Check sheet for the modelled part. Datum: model origin and axes. Units: mm. Face numbers are marked on the shaded views. A direction names the side the tool comes from. Round coordinates to 2 decimals unless told otherwise and drop trailing zeros. Write each loop counter-clockwise with the first axis right and the second up, starting at its lowest first coordinate (ties: lowest second). Pieces come first, ordered by that corner, then holes. Notation, with made-up numbers: (-26, 64) -> (-9, 64) arc R25 ccw to (-9, 82) -> close; hole circle Ø8 at (77.5, 32). An arc over 180 degrees is marked (long way). Answer as a JSON object with one key per item and string values. Group by question number.
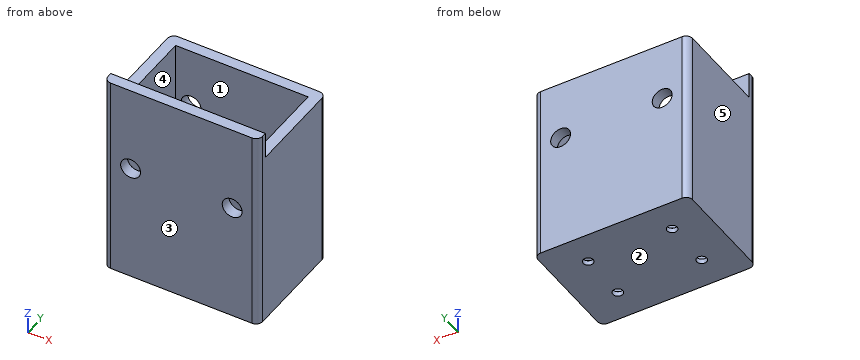
```python
from build123d import *

# Parameters (mm, degrees)
SKETCH1_W                                   = 70
SKETCH1_H                                   = 50
BOSS_EXTRUDE1_DEPTH                         = 5
SKETCH2_W                                   = 70
SKETCH2_H                                   = 5
BOSS_EXTRUDE2_DEPTH                         = 88
BOSS_EXTRUDE3_DEPTH                         = 76
SKETCH4_R                                   = 4.5
CUT_EXTRUDE1_DEPTH                          = 56
FILLET1_R                                   = 3
CBORE_FOR_M4_HEX_HEAD_CAP_SCREW1_AT_2_COUNT = 2
CBORE_FOR_M4_HEX_HEAD_CAP_SCREW1_AT_2_PITCH = 22
CBORE_FOR_M4_HEX_HEAD_CAP_SCREW1_AT_3_COUNT = 2
CBORE_FOR_M4_HEX_HEAD_CAP_SCREW1_AT_3_PITCH = 43.9089968
CBORE_FOR_M4_HEX_HEAD_CAP_SCREW1_AT_4_COUNT = 2
CBORE_FOR_M4_HEX_HEAD_CAP_SCREW1_AT_4_PITCH = 38


with BuildPart() as part:
    # Sketch1 → Boss-Extrude1 (new body)
    with BuildSketch(Plane.XY):
        Rectangle(SKETCH1_W, SKETCH1_H)
    extrude(amount=BOSS_EXTRUDE1_DEPTH)

    # Sketch2 → Boss-Extrude2 (add)
    with BuildSketch(Plane.XY.offset(5)):
        with Locations((0, -22.5)):
            Rectangle(SKETCH2_W, SKETCH2_H)
    extrude(amount=BOSS_EXTRUDE2_DEPTH)

    # Sketch3 → Boss-Extrude3 (add)
    with BuildSketch(Plane.XY.offset(5)):
        Polygon((-35, 25), (35, 25), (35, 20), (35, -20), (30, -20), (30, 20), (-30, 20), (-30, -20), (-35, -20), (-35, 20), align=None)
    extrude(amount=BOSS_EXTRUDE3_DEPTH)

    # Sketch4 → Cut-Extrude1 (cut)
    with BuildSketch(Plane(origin=(0, 25, 0), x_dir=(1, 0, 0), z_dir=(0, 1, 0))):
        with Locations(Location((23, -54, 0), (0, 0, 270))):
            Circle(SKETCH4_R)
        with Locations(Location((-23, -54, 0), (0, 0, 270))):
            Circle(SKETCH4_R)
    extrude(amount=-CUT_EXTRUDE1_DEPTH, mode=Mode.SUBTRACT)

    # Fillet1
    fillet1_edges = [part.edges().sort_by_distance(p)[0] for p in [
        (-35, 25, 40.5),
        (35, 25, 40.5),
        (35, -25, 46.5),
        (-35, -25, 46.5),
    ]]
    fillet(fillet1_edges, radius=FILLET1_R)

    # Sketch7 → CBORE for M4 Hex Head Cap Screw1 (revolve, cut)
    with BuildSketch(Plane(origin=(-19, -11, 5), x_dir=(0, -1, 0), z_dir=(1, 0, 0))):
        Polygon((0, 0), (0, 12.4), (2.25, 11.048063607), (2.25, 2.8), (5.5415, 2.8), (5.5415, 0.025), (5.5665, 0), align=None)
    cbore_for_m4_hex_head_cap_screw1 = revolve(axis=Axis((-19, -11, 11.35), (0, 0, -1)), mode=Mode.SUBTRACT)

    # CBORE for M4 Hex Head Cap Screw1 at 2: CBORE for M4 Hex Head Cap Screw1 ×2
    with Locations(*[(0, i * CBORE_FOR_M4_HEX_HEAD_CAP_SCREW1_AT_2_PITCH, 0) for i in range(1, CBORE_FOR_M4_HEX_HEAD_CAP_SCREW1_AT_2_COUNT)]):
        add(cbore_for_m4_hex_head_cap_screw1, mode=Mode.SUBTRACT)

    # CBORE for M4 Hex Head Cap Screw1 at 3: CBORE for M4 Hex Head Cap Screw1 ×2
    with Locations(*[Vector(0.8654262854811263, 0.5010362705417046, 0) * (i * CBORE_FOR_M4_HEX_HEAD_CAP_SCREW1_AT_3_PITCH) for i in range(1, CBORE_FOR_M4_HEX_HEAD_CAP_SCREW1_AT_3_COUNT)]):
        add(cbore_for_m4_hex_head_cap_screw1, mode=Mode.SUBTRACT)

    # CBORE for M4 Hex Head Cap Screw1 at 4: CBORE for M4 Hex Head Cap Screw1 ×2
    with Locations(*[(i * CBORE_FOR_M4_HEX_HEAD_CAP_SCREW1_AT_4_PITCH, 0, 0) for i in range(1, CBORE_FOR_M4_HEX_HEAD_CAP_SCREW1_AT_4_COUNT)]):
        add(cbore_for_m4_hex_head_cap_screw1, mode=Mode.SUBTRACT)


solid = part.part
```
(1) Go/stop test with flat-tipped pins: pin 1 Ø12 at (x, y) = (20.5, -12.5) entering from +Z; pin 2 Ø9 at (x, y) = (19, -11) entering from -Z; pin 3 Ø3.5 at (x, y) = (-16.5, 9) entering from +Z. Record where each tip stops, or that it passes through.
(2) Section check B-B on z = 54. Record the cut outline in (x, y).
(3) Release check for a two-part mould opening along Y. For the marked faces 3, 4 and 5 record: pulls with the +Y half, pulls with the -Y half, needs draft (parallel to the pull), parting line crosses it, or undercut.
(4) Section check C-C on x = -12. Record the cut outline in (y, z), then the cut area to 3 significant figures.
(5) Section check A-A on y = -11. State how many separate pieces and enclosed holes the cut face has, then the cut area to 3 significant figures.
(6) Scan lines: line 1 along X through (y, z) = (-11, 3.7); line 2 along Y through (x, z) = (-19, 3.4); line 3 along X through (y, z) = (22.2, 54). Record each from-to range of solid material in increasing order.
(7) Section check D-D on y = 3. Record the cut outline in (x, z), then the cut area to 3 significant figures.
(8) Access from +Z, -Z, +X, -X, +Y, -Y to the whole of each face (thin tool, end or side, straight path). Record for the marked faces 1 and 2.
Data:
{
 "1": {"pin 1": "stops at z = 5", "pin 2": "stops at z = 0", "pin 3": "stops at z = 2.2"},
 "2": {"outline": "(-35, -22) arc R3 ccw to (-32, -25) -> (-27.5, -25) -> (-27.5, -20) -> (-30, -20) -> (-30, 20) -> (-27.5, 20) -> (-27.5, 25) -> (-32, 25) arc R3 ccw to (-35, 22) -> close; (-18.5, -25) -> (18.5, -25) -> (18.5, -20) -> (-18.5, -20) -> close; (-18.5, 20) -> (18.5, 20) -> (18.5, 25) -> (-18.5, 25) -> close; (27.5, -25) -> (32, -25) arc R3 ccw to (35, -22) -> (35, 22) arc R3 ccw to (32, 25) -> (27.5, 25) -> (27.5, 20) -> (30, 20) -> (30, -20) -> (27.5, -20) -> close"},
 "3": {"face 3": "pulls with the -Y half", "face 4": "undercut", "face 5": "needs draft"},
 "4": {"outline": "(-25, 0) -> (25, 0) -> (25, 81) -> (20, 81) -> (20, 5) -> (-20, 5) -> (-20, 93) -> (-25, 93) -> close", "area": "1,070 mm²"},
 "5": {"separate pieces": "3", "enclosed holes": "0", "area": "1,030 mm²"},
 "6": {"line 1": "x = -35 to -24.54, -13.46 to 13.46, 24.54 to 35", "line 2": "y = -25 to -16.54, -5.46 to 5.46, 16.54 to 25", "line 3": "x = -34.99 to -27.5, -18.5 to 18.5, 27.5 to 34.99"},
 "7": {"outline": "(-35, 0) -> (35, 0) -> (35, 81) -> (30, 81) -> (30, 5) -> (-30, 5) -> (-30, 81) -> (-35, 81) -> close", "area": "1,110 mm²"},
 "8": {"face 1": "+Z", "face 2": "-Z, +X, -X, +Y, -Y"}
}
